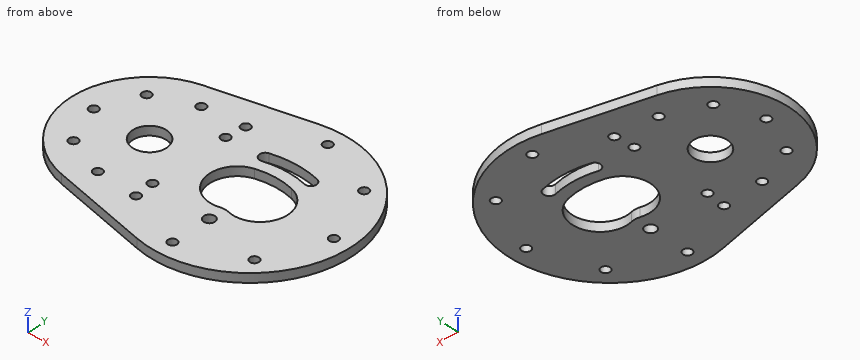
```python
from build123d import *

# Parameters (mm, degrees)
SKETCH1_W           = 127
SKETCH1_H           = 88.9
SKETCH1_R           = 1.564880276
SKETCH1_R_2         = 4.7625
BOSS_EXTRUDE1_DEPTH = 2.54
SKETCH2_W           = 177.519600035
SKETCH2_H           = 126.718171086
CUT_EXTRUDE1_DEPTH  = 108.831991492
SKETCH4_R           = 1.27
CUT_EXTRUDE2_DEPTH  = 66.377727285


with BuildPart() as part:
    # Sketch1 → Boss-Extrude1 (new body)
    with BuildSketch(Plane.XY):
        with Locations((-28.03132955, 12.5)):
            Rectangle(SKETCH1_W, SKETCH1_H)
        Circle(SKETCH1_R, mode=Mode.SUBTRACT)
        with Locations((-28.575, 12.5)):
            Circle(SKETCH1_R_2, mode=Mode.SUBTRACT)
        with BuildLine():
            ThreePointArc((5.250170212, 19.593901979), (10.755067214, 10.059140681), (1.220305916, 4.554243678))
            ThreePointArc((1.220305916, 4.554243678), (0, 4.7149), (-1.220305916, 4.554243678))
            ThreePointArc((-1.220305916, 4.554243678), (-10.755067214, 10.059140681), (-5.250170212, 19.593901979))
            ThreePointArc((-5.250170212, 19.593901979), (0, 20.2851), (5.250170212, 19.593901979))
        make_face(mode=Mode.SUBTRACT)
        with BuildLine():
            ThreePointArc((6.881351362, 25.681552906), (0, 26.5875), (-6.881351362, 25.681552906))
            ThreePointArc((-6.881351362, 25.681552906), (-8.003883377, 23.737270423), (-6.059600893, 22.614738408))
            ThreePointArc((-6.059600893, 22.614738408), (0, 23.4125), (6.059600893, 22.614738408))
            ThreePointArc((6.059600893, 22.614738408), (8.003883377, 23.737270423), (6.881351362, 25.681552906))
        make_face(mode=Mode.SUBTRACT)
    extrude(amount=BOSS_EXTRUDE1_DEPTH)

    # Sketch2 → Cut-Extrude1 (cut, through all)
    with BuildSketch(Plane.XY.offset(2.54)):
        with Locations((-18.257651528, 17.008273159)):
            Rectangle(SKETCH2_W, SKETCH2_H)
        with BuildLine():
            Line((-33.513888889, 34.169287057), (-6.35, 40.36051193))
            ThreePointArc((-6.35, 40.36051193), (28.575, 12.5), (-6.35, -15.36051193))
            Line((-6.35, -15.36051193), (-33.513888889, -9.169287057))
            ThreePointArc((-33.513888889, -9.169287057), (-50.8, 12.5), (-33.513888889, 34.169287057))
        make_face(mode=Mode.SUBTRACT)
    extrude(amount=-CUT_EXTRUDE1_DEPTH, mode=Mode.SUBTRACT)

    # Sketch4 → Cut-Extrude2 (cut, through all)
    with BuildSketch(Plane.XY.offset(2.54)):
        with Locations((-28.575, 28.375)):
            Circle(SKETCH4_R)
        with Locations((0, 36.3125)):
            Circle(SKETCH4_R)
        with Locations((-17.349679849, 23.725320151)):
            Circle(SKETCH4_R)
        with Locations((-17.349679849, 1.274679849)):
            Circle(SKETCH4_R)
        with Locations((-28.575, -3.375)):
            Circle(SKETCH4_R)
        with Locations((-39.800320151, 1.274679849)):
            Circle(SKETCH4_R)
        with Locations((-44.45, 12.5)):
            Circle(SKETCH4_R)
        with Locations((-39.800320151, 23.725320151)):
            Circle(SKETCH4_R)
        with Locations((16.837980227, 29.337980227)):
            Circle(SKETCH4_R)
        with Locations((23.8125, 12.5)):
            Circle(SKETCH4_R)
        with Locations((16.837980227, -4.337980227)):
            Circle(SKETCH4_R)
        with Locations((0, -11.3125)):
            Circle(SKETCH4_R)
        with Locations((-16.837980227, -4.337980227)):
            Circle(SKETCH4_R)
        with Locations((-16.837980227, 29.337980227)):
            Circle(SKETCH4_R)
    extrude(amount=-CUT_EXTRUDE2_DEPTH, mode=Mode.SUBTRACT)


solid = part.part
```
The model under review builds one solid part; all positions refer to its coordinate system, in mm. Coordinates: 2 decimals unless noted, no trailing zeros. Write each loop counter-clockwise with the first axis right and the second up, starting at its lowest first coordinate (ties: lowest second). Pieces come first, ordered by that corner, then holes. Notation, with made-up numbers: (66.25, 5) -> (84.25, 5) arc R25 cw to (84.25, 25) -> close; hole circle Ø10 at (59.5, 79). An arc over 180 degrees is marked (long way). One line per item, written item: value. Start each with the question number.
Q1. Clearance check with a flat-ended pin moving along its axis: P1, Ø1, axis at x = -29, z = 1.5, coming from the -Y side. State where the tip first meets the part, or that it passes through.
Q2. Add section D-D, the plane z = 0.4. Count the separate pieces of the cut face and the enclosed holes in it, then the cut area to 3 significant figures.
Q3. Add section B-B, the plane y = 12.5. Give the boundary of the cut face in (x, z) (1 decimal).
Q4. To check wall thickness, follow probe 1 along X at (y, z) = (13.5, 1.3); probe 2 along Y at (x, z) = (-39, 2.1); probe 3 along Y at (x, z) = (17, 0.8). State the ranges of each line that lie inside material, in increasing order.
Q5. Add section C-C, the plane x = -40. Give the boundary of the cut face in (y, z), then the cut area to 3 significant figures.
Q6. Add section A-A, the plane x = 0. Give the boundary of the cut face in (y, z) (1 decimal), then the cut area to 3 significant figures.
Response:
1. P1: y = -10.31
2. separate pieces: 1
2. enclosed holes: 18
2. area: 3,050 mm²
3. outline: (-50.8, 0) -> (-45.7, 0) -> (-45.7, 2.5) -> (-50.8, 2.5) -> close; (-43.2, 0) -> (-33.3, 0) -> (-33.3, 2.5) -> (-43.2, 2.5) -> close; (-23.8, 0) -> (-11, 0) -> (-11, 2.5) -> (-23.8, 2.5) -> close; (11, 0) -> (22.5, 0) -> (22.5, 2.5) -> (11, 2.5) -> close; (25.1, 0) -> (28.6, 0) -> (28.6, 2.5) -> (25.1, 2.5) -> close
4. probe 1: -50.78 to -45.23, -43.67 to -33.23, -23.92 to -10.89, 10.89 to 23.03, 24.6 to 28.56
4. probe 2: -7.13 to 0.29, 2.26 to 22.74, 24.71 to 32.13
4. probe 3: -10.47 to -5.6, -3.08 to 28.08, 30.6 to 35.47
5. outline: (-6.56, 0) -> (0.02, 0) -> (0.02, 2.54) -> (-6.56, 2.54) -> close; (2.53, 0) -> (22.47, 0) -> (22.47, 2.54) -> (2.53, 2.54) -> close; (24.98, 0) -> (31.56, 0) -> (31.56, 2.54) -> (24.98, 2.54) -> close
5. area: 84.1 mm²
6. outline: (-16.1, 0) -> (-12.6, 0) -> (-12.6, 2.5) -> (-16.1, 2.5) -> close; (-10, 0) -> (-1.6, 0) -> (-1.6, 2.5) -> (-10, 2.5) -> close; (1.6, 0) -> (4.7, 0) -> (4.7, 2.5) -> (1.6, 2.5) -> close; (20.3, 0) -> (23.4, 0) -> (23.4, 2.5) -> (20.3, 2.5) -> close; (26.6, 0) -> (35, 0) -> (35, 2.5) -> (26.6, 2.5) -> close; (37.6, 0) -> (41.1, 0) -> (41.1, 2.5) -> (37.6, 2.5) -> close
6. area: 76.7 mm²
